The model under review builds one solid part; all positions refer to its coordinate system, in mm. Face numbers are marked on the shaded views. A direction names the side the tool comes from. Give positions to 0.01 mm unless a question says otherwise; leave off trailing zeros. Order: outer loops, then holes, each group sorted by start corner. A loop starts at its lowest first (then second) coordinate and runs counter-clockwise, first axis right, second up.
```python
from build123d import *

# Parameters (mm, degrees)
F0_R     = 19.05
F0_R_2   = 4.7625
F1_DEPTH = 25.4
F2_DEPTH = 50.8
F4_R     = 12.7
F3_R     = 25.8953
F5_DEPTH = 19.051
F6_DEPTH = 25.4
F7_ANGLE = 90


with BuildPart() as f1:
    # F0 (on Top) → F1 (new body)
    with BuildSketch(Plane.XY):
        Circle(F0_R)
        Circle(F0_R_2, mode=Mode.SUBTRACT)
    extrude(amount=F1_DEPTH)

    # F0 (on Top) → F2 (join)
    with BuildSketch(Plane.XY):
        Circle(F0_R_2)
    extrude(amount=F2_DEPTH)

    # F4
    f4_edges = [f1.edges().sort_by_distance(p)[0] for p in [
        (-19.05, 0, 0),
    ]]
    fillet(f4_edges, radius=F4_R)

    # F3 (on Front) → F5 (cut, through all)
    with BuildSketch(Plane.XZ):
        with Locations((19.05, 0)):
            Circle(F3_R)
    extrude(amount=-F5_DEPTH, mode=Mode.SUBTRACT)

    # F3 (on Front) → F6 (cut)
    with BuildSketch(Plane.XZ):
        with Locations((19.05, 0)):
            Circle(F3_R)
    extrude(amount=F6_DEPTH, mode=Mode.SUBTRACT)


with BuildPart() as f1_1:
    # F7: moved
    add(f1.part.rotate(Axis((0, 0, 0), (0, 0, -1)), F7_ANGLE))


solid = f1_1.part
```
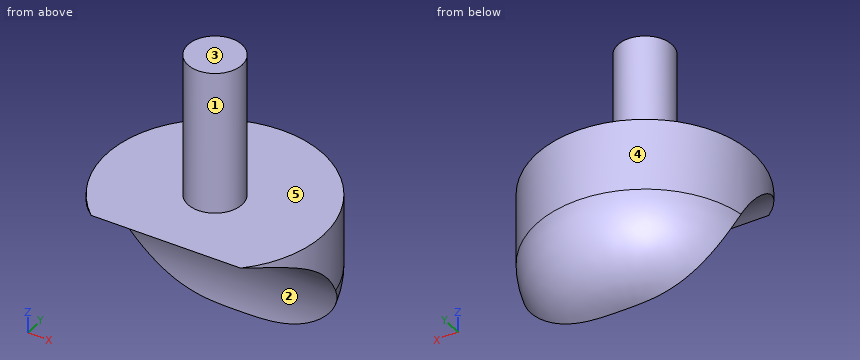
1. Take a section at B-B (z = 15). Write out the cut boundary in (x, y).
2. Insertion check: pin 1 (12 mm diameter, centred on y = -1, z = 43.5, fed in from +X); pin 2 (4 mm diameter, centred on x = -9, y = 13.5, fed in from +Z); pin 3 (8 mm diameter, centred on y = 0.5, z = 41.5, fed in from -X). Each pin has a flat end and moves straight along its axis. Give the tip position at first contact, or say it passes through.
3. Take a section at A-A (y = 0). Write out the cut boundary in (x, z), and give its area (3 significant figures).
4. To check wall thickness, follow line 1 (Z direction, x = 3.5, y = 16.5); line 2 (Z direction, x = -1, y = 7); line 3 (X direction, y = 1.5, z = 48.5). State the ranges of each line that lie inside material, in increasing order.
5. For the marked faces 4 and 5, list the 3-axis set-ups (+Z, -Z, +X, -X, +Y, -Y) from which the entire face can be reached by the end or side of a thin tool; tool diameter is ignored.
6. Draft analysis for pull direction Z (two halves, no side actions). For the marked faces 1, 2 and 3, state which applies: pulls with the +Z half, pulls with the -Z half, needs draft (parallel to the pull), parting line crosses it, or undercut.
Answer:
1. outline: (-18.94, 2.06) - (18.94, 2.06) arc R19.05 ccw to start
2. pin 1: stops at x = 4.76
2. pin 2: stops at z = 25.4
2. pin 3: stops at x = -4.76
3. outline: (-19.05, 17.54) - (19.05, 17.54) - (19.05, 25.4) - (4.76, 25.4) - (4.76, 50.8) - (-4.76, 50.8) - (-4.76, 25.4) - (-19.05, 25.4) - close
3. area: 541 mm2
4. line 1: z = 5.58 to 25.4
4. line 2: z = 0.02 to 25.4
4. line 3: x = -4.52 to 4.52
5. face 4: +Z, -Z
5. face 5: +Z
6. face 1: needs draft
6. face 2: pulls with the -Z half
6. face 3: pulls with the +Z half
